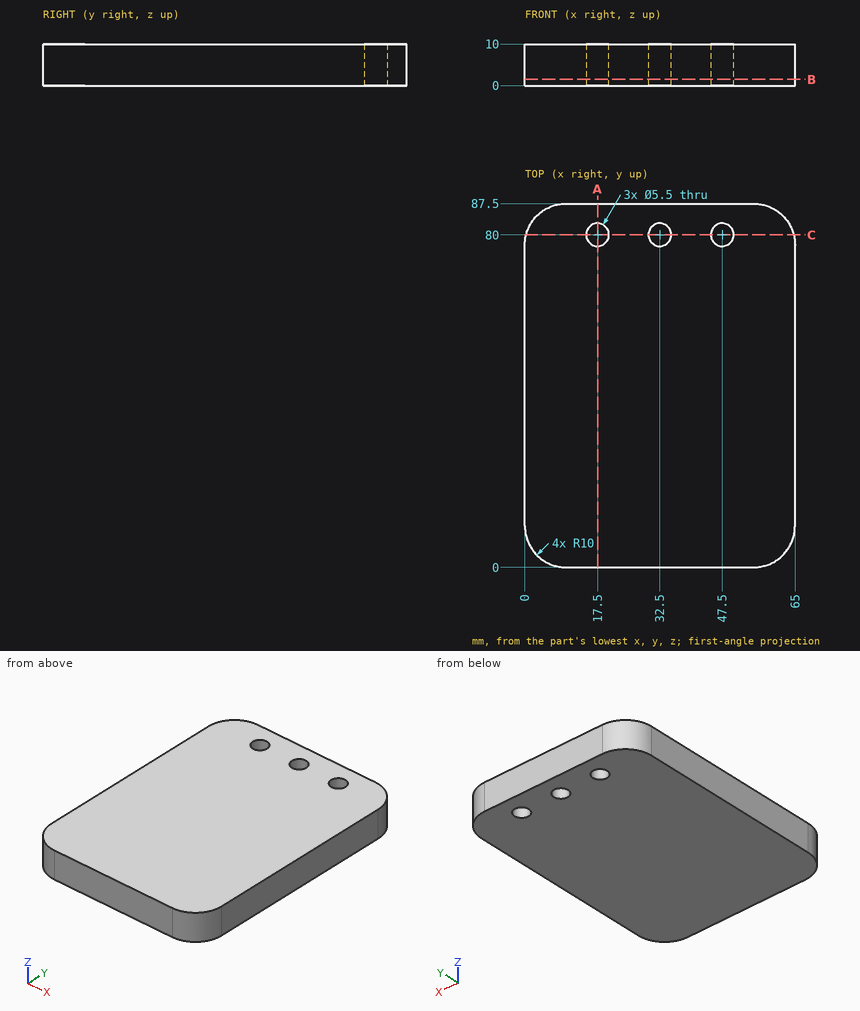
Print and shaded views of the part. All mm, measured from the part's lowest x, y and z. Round coordinates to 2 decimals unless told otherwise and drop trailing zeros. Loops run counter-clockwise (first coordinate to the right, second up) from the corner with the lowest first, then second, coordinate; pieces in that order, holes last. Notation, with made-up numbers: M 18,60 L 44,60 A10 ccw 44,72 Z; hole C 43,63.25 d1. An arc over 180 degrees is marked long. One line per question, with ' | ' between items.
1) Flat gauge pins, fed straight in: pin 1 (6 mm diameter, centred on x = 19, y = 78, fed in from -Z); pin 2 (4.5 mm diameter, centred on x = 47.5, y = 80, fed in from -Z) (1 decimal). Where does each tip first touch, or does it go through?
Solved:
pin 1: stops at z = 0 | pin 2: passes through
2) Drill centre lines: line 1 along Y through (x, z) = (32.5, 5); line 2 along X through (y, z) = (80, 6); line 3 along Y through (x, z) = (15, 4.75). Where is each one in solid material? Low to high.
Solved:
line 1: y = 0 to 77.25, 82.75 to 87.5 | line 2: x = 0.32 to 14.75, 20.25 to 29.75, 35.25 to 44.75, 50.25 to 64.68 | line 3: y = 0 to 78.85, 81.15 to 87.5
3) Band-saw the part on B-B (z = 1.5). Give the cut face in (x, y), then the cut area to 3 significant figures.
Solved:
outline: M 0,10 A10 ccw 10,0 L 55,0 A10 ccw 65,10 L 65,77.5 A10 ccw 55,87.5 L 10,87.5 A10 ccw 0,77.5 Z; hole C 17.5,80 d5.5; hole C 32.5,80 d5.5; hole C 47.5,80 d5.5 | area: 5,530 mm²
4) Band-saw the part on A-A (x = 17.5). Give the cut face in (y, z).
Solved:
outline: M 0,0 L 77.25,0 L 77.25,10 L 0,10 Z; M 82.75,0 L 87.5,0 L 87.5,10 L 82.75,10 Z
5) Band-saw the part on C-C (y = 80). Give the cut face in (x, z).
Solved:
outline: M 0.32,0 L 14.75,0 L 14.75,10 L 0.32,10 Z; M 20.25,0 L 29.75,0 L 29.75,10 L 20.25,10 Z; M 35.25,0 L 44.75,0 L 44.75,10 L 35.25,10 Z; M 50.25,0 L 64.68,0 L 64.68,10 L 50.25,10 Z
